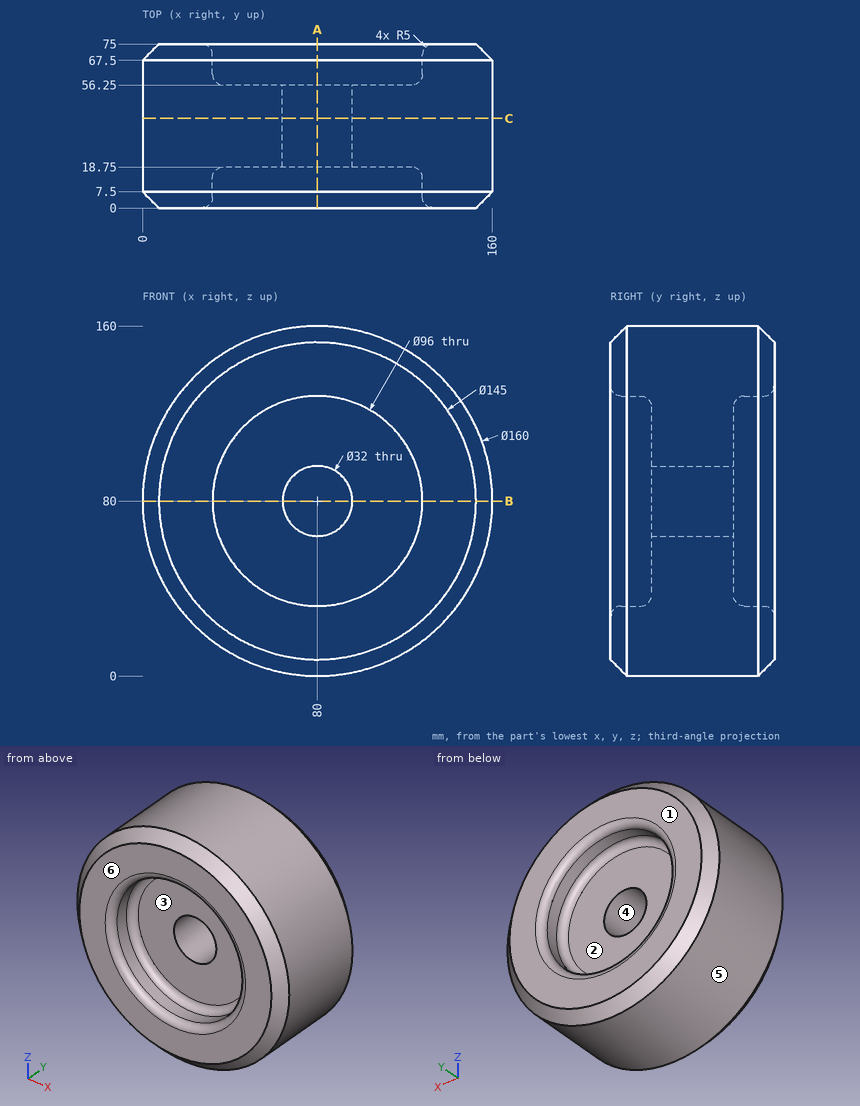
Drawing for the job (mm, zero at the part's lowest x, y, z). A direction names the side the tool comes from. Round coordinates to 2 decimals unless told otherwise and drop trailing zeros. Order: outer loops, then holes, each group sorted by start corner. A loop starts at its lowest first (then second) coordinate and runs counter-clockwise, first axis right, second up.
Item 1: Pin check, flat tips, straight feed: pin 1 (4 mm diameter, centred on x = 91.5, z = 101, fed in from -Y); pin 2 (5 mm diameter, centred on x = 126, z = 78, fed in from -Y); pin 3 (1 mm diameter, centred on y = 13, z = 64.5, fed in from -X). Stop position of each tip, or through.
Item 2: Probe line 1 along Z through (x, y) = (79, 26.5); line 2 along Z through (x, y) = (80, 63); line 3 along Y through (x, z) = (109, 104.5). List the from-to ranges inside material, lowest first.
Item 3: Saw through at A-A on x = 80. Write the cut outline in (y, z), then the cut area to 3 significant figures.
Item 4: Mould opens along Z. For the marked faces 4, 5 and 6 say: pulls with the +Z half, pulls with the -Z half, needs draft (parallel to the pull), parting line crosses it, or undercut.
Item 5: Tool access for the marked faces 1, 2 and 3: list every direction of +Z, -Z, +X, -X, +Y, -Y with a clear straight run to the whole face (end or side of a thin tool).
Item 6: Saw through at C-C on y = 41. Write the cut outline in (x, z), then the cut area to 3 significant figures.
Item 7: Saw through at B-B on z = 80. Write the cut outline in (x, y), then the cut area to 3 significant figures.
Reported:
1. pin 1: stops at y = 18.75
1. pin 2: stops at y = 2.73
1. pin 3: stops at x = 1.42
2. line 1: z = 0.01 to 64.03, 95.97 to 159.99
2. line 2: z = 0 to 32, 128 to 160
2. line 3: y = 18.75 to 56.25
3. outline: (0, 7.5) - (7.5, 0) - (67.5, 0) - (75, 7.5) - (75, 27) arc R5 ccw to (70, 32) - (61.25, 32) arc R5 cw to (56.25, 37) - (56.25, 64) - (18.75, 64) - (18.75, 37) arc R5 cw to (13.75, 32) - (5, 32) arc R5 ccw to (0, 27) - close; (0, 133) arc R5 ccw to (5, 128) - (13.75, 128) arc R5 cw to (18.75, 123) - (18.75, 96) - (56.25, 96) - (56.25, 123) arc R5 cw to (61.25, 128) - (70, 128) arc R5 ccw to (75, 133) - (75, 152.5) - (67.5, 160) - (7.5, 160) - (0, 152.5) - close
3. area: 7,090 mm2
4. face 4: undercut
4. face 5: parting line crosses it
4. face 6: needs draft
5. face 1: +Z, -Z, +X, -X, +Y
5. face 2: +Y
5. face 3: -Y
6. outline: circle Ø160 at (80, 80); hole circle Ø32 at (80, 80)
6. area: 19,300 mm2
7. outline: (0, 7.5) - (7.5, 0) - (27, 0) arc R5 ccw to (32, 5) - (32, 13.75) arc R5 cw to (37, 18.75) - (64, 18.75) - (64, 56.25) - (37, 56.25) arc R5 cw to (32, 61.25) - (32, 70) arc R5 ccw to (27, 75) - (7.5, 75) - (0, 67.5) - close; (96, 18.75) - (123, 18.75) arc R5 cw to (128, 13.75) - (128, 5) arc R5 ccw to (133, 0) - (152.5, 0) - (160, 7.5) - (160, 67.5) - (152.5, 75) - (133, 75) arc R5 ccw to (128, 70) - (128, 61.25) arc R5 cw to (123, 56.25) - (96, 56.25) - close
7. area: 7,090 mm2
